Source: CAD feature listing. Evaluate the final solid. Frame: model axes, mm. A direction names the side the tool comes from. Coordinates: 2 decimals unless noted, no trailing zeros. Order: outer loops, then holes, each group sorted by start corner. A loop starts at its lowest first (then second) coordinate and runs counter-clockwise, first axis right, second up.
```python
from build123d import *

# Parameters (mm, degrees)
SKETCH1_W                                      = 25.4
SKETCH1_H                                      = 29
BOSS_EXTRUDE1_DEPTH                            = 8
SKETCH2_W                                      = 275
SKETCH2_H                                      = 29
BOSS_EXTRUDE2_DEPTH                            = 7
CBORE_FOR_8_SOCKET_HEAD_CAP_SCREW1_D           = 4.4958
CBORE_FOR_8_SOCKET_HEAD_CAP_SCREW1_DEPTH       = 18.649325414
CBORE_FOR_8_SOCKET_HEAD_CAP_SCREW1_CBORE_D     = 7.9375
CBORE_FOR_8_SOCKET_HEAD_CAP_SCREW1_CBORE_DEPTH = 4.1656
CBORE_FOR_8_SOCKET_HEAD_CAP_SCREW1_TIP         = 1.350674586
SKETCH5_W                                      = 64.25
SKETCH5_H                                      = 10.5
SKETCH5_W_2                                    = 109.45
SKETCH5_W_3                                    = 11.4
SKETCH5_W_4                                    = 6.7
CUT_EXTRUDE1_DEPTH                             = 10
FILLET1_R                                      = 3.9
FILLET2_R                                      = 3.5


with BuildPart() as part:
    # Sketch1 → Boss-Extrude1 (new body)
    with BuildSketch(Plane.XY):
        Rectangle(SKETCH1_W, SKETCH1_H)
    extrude(amount=BOSS_EXTRUDE1_DEPTH)

    # Sketch2 → Boss-Extrude2 (add)
    with BuildSketch(Plane.XY.offset(8)):
        with Locations((124.8, 0)):
            Rectangle(SKETCH2_W, SKETCH2_H)
    extrude(amount=BOSS_EXTRUDE2_DEPTH)

    # CBORE for #8 Socket Head Cap Screw1
    with Locations(Plane(origin=(-7.5, 7.5, 15), x_dir=(1, 0, 0), z_dir=(0, 0, 1))):
        with Locations((0, 0), (15, 0), (15, -15), (0, -15), (35.7, 0), (35.7, -15), (113.95, 0), (113.95, -15), (237.4, 0), (237.4, -15), (262.8, 0), (262.8, -15)):
            CounterBoreHole(CBORE_FOR_8_SOCKET_HEAD_CAP_SCREW1_D / 2, CBORE_FOR_8_SOCKET_HEAD_CAP_SCREW1_CBORE_D / 2, CBORE_FOR_8_SOCKET_HEAD_CAP_SCREW1_CBORE_DEPTH, depth=CBORE_FOR_8_SOCKET_HEAD_CAP_SCREW1_DEPTH)
            with Locations((0, 0, -(CBORE_FOR_8_SOCKET_HEAD_CAP_SCREW1_DEPTH + CBORE_FOR_8_SOCKET_HEAD_CAP_SCREW1_TIP / 2))):  # 118° drill point
                Cone(0, CBORE_FOR_8_SOCKET_HEAD_CAP_SCREW1_D / 2, CBORE_FOR_8_SOCKET_HEAD_CAP_SCREW1_TIP, mode=Mode.SUBTRACT)

    # Sketch5 → Cut-Extrude1 (cut)
    with BuildSketch(Plane.XY.offset(15)):
        with Locations((67.325, 9.25)):
            Rectangle(SKETCH5_W, SKETCH5_H)
        with Locations((168.175, 9.25)):
            Rectangle(SKETCH5_W_2, SKETCH5_H)
        with Locations((242.6, 9.25)):
            Rectangle(SKETCH5_W_3, SKETCH5_H)
        with Locations((17.85, 9.25)):
            Rectangle(SKETCH5_W_4, SKETCH5_H)
    cut_extrude1 = extrude(amount=-CUT_EXTRUDE1_DEPTH, mode=Mode.SUBTRACT)

    # Mirror1: Cut-Extrude1 across plane
    add(cut_extrude1.mirror(Plane.ZX), mode=Mode.SUBTRACT)

    # Fillet1
    # the kernel refuses this fillet: 3.9 mm, written as the material it takes off along each edge
    with BuildSketch(Plane(origin=(222.9, 4, 15), x_dir=(0, -1, 0), z_dir=(-1, 0, 0)), Plane(origin=(222.9, -4, 8), x_dir=(0, 1, 0), z_dir=(-1, 0, 0))) as fillet1_piece_1:
        with BuildLine():
            CenterArc((FILLET1_R, -FILLET1_R), FILLET1_R, 90, 90)
            Line((0, -FILLET1_R), (0, 0))
            Line((0, 0), (FILLET1_R, 0))
        make_face()
    extrude(amount=109.45, mode=Mode.SUBTRACT)
    with BuildSketch(Plane(origin=(248.3, 4, 15), x_dir=(0, -1, 0), z_dir=(-1, 0, 0)), Plane(origin=(248.3, -4, 8), x_dir=(0, 1, 0), z_dir=(-1, 0, 0))) as fillet1_piece_2:
        with BuildLine():
            CenterArc((FILLET1_R, -FILLET1_R), FILLET1_R, 90, 90)
            Line((0, -FILLET1_R), (0, 0))
            Line((0, 0), (FILLET1_R, 0))
        make_face()
    extrude(amount=11.4, mode=Mode.SUBTRACT)
    with BuildSketch(Plane(origin=(248.3, 4, 8), x_dir=(0, -1, 0), z_dir=(-1, 0, 0)), Plane(origin=(248.3, -4, 15), x_dir=(0, 1, 0), z_dir=(-1, 0, 0))) as fillet1_piece_3:
        with BuildLine():
            CenterArc((FILLET1_R, FILLET1_R), FILLET1_R, 180, 90)
            Line((0, FILLET1_R), (0, 0))
            Line((0, 0), (FILLET1_R, 0))
        make_face()
    extrude(amount=11.4, mode=Mode.SUBTRACT)
    with BuildSketch(Plane(origin=(222.9, -4, 15), x_dir=(0, 1, 0), z_dir=(-1, 0, 0)), Plane(origin=(222.9, 4, 8), x_dir=(0, -1, 0), z_dir=(-1, 0, 0))) as fillet1_piece_4:
        with BuildLine():
            CenterArc((FILLET1_R, FILLET1_R), FILLET1_R, 180, 90)
            Line((0, FILLET1_R), (0, 0))
            Line((0, 0), (FILLET1_R, 0))
        make_face()
    extrude(amount=109.45, mode=Mode.SUBTRACT)
    with BuildSketch(Plane(origin=(99.45, 4, 8), x_dir=(0, -1, 0), z_dir=(-1, 0, 0)), Plane(origin=(99.45, -4, 15), x_dir=(0, 1, 0), z_dir=(-1, 0, 0))) as fillet1_piece_5:
        with BuildLine():
            CenterArc((FILLET1_R, FILLET1_R), FILLET1_R, 180, 90)
            Line((0, FILLET1_R), (0, 0))
            Line((0, 0), (FILLET1_R, 0))
        make_face()
    extrude(amount=64.25, mode=Mode.SUBTRACT)
    with BuildSketch(Plane(origin=(99.45, 4, 15), x_dir=(0, -1, 0), z_dir=(-1, 0, 0)), Plane(origin=(99.45, -4, 8), x_dir=(0, 1, 0), z_dir=(-1, 0, 0))) as fillet1_piece_6:
        with BuildLine():
            CenterArc((FILLET1_R, -FILLET1_R), FILLET1_R, 90, 90)
            Line((0, -FILLET1_R), (0, 0))
            Line((0, 0), (FILLET1_R, 0))
        make_face()
    extrude(amount=64.25, mode=Mode.SUBTRACT)
    with BuildSketch(Plane(origin=(21.2, -4, 8), x_dir=(0, 1, 0), z_dir=(-1, 0, 0)), Plane(origin=(21.2, 4, 15), x_dir=(0, -1, 0), z_dir=(-1, 0, 0))) as fillet1_piece_7:
        with BuildLine():
            CenterArc((FILLET1_R, -FILLET1_R), FILLET1_R, 90, 90)
            Line((0, -FILLET1_R), (0, 0))
            Line((0, 0), (FILLET1_R, 0))
        make_face()
    extrude(amount=6.7, mode=Mode.SUBTRACT)
    with BuildSketch(Plane(origin=(21.2, -4, 15), x_dir=(0, 1, 0), z_dir=(-1, 0, 0)), Plane(origin=(21.2, 4, 8), x_dir=(0, -1, 0), z_dir=(-1, 0, 0))) as fillet1_piece_8:
        with BuildLine():
            CenterArc((FILLET1_R, FILLET1_R), FILLET1_R, 180, 90)
            Line((0, FILLET1_R), (0, 0))
            Line((0, 0), (FILLET1_R, 0))
        make_face()
    extrude(amount=6.7, mode=Mode.SUBTRACT)

    # Fillet2
    fillet2_edges = [part.edges().sort_by_distance(p)[0] for p in [
        (262.3, -14.5, 11.5),
        (14.5, 14.5, 11.5),
        (21.2, 14.5, 11.5),
        (262.3, 14.5, 11.5),
        (236.9, 14.5, 11.5),
        (248.3, 14.5, 11.5),
        (113.45, 14.5, 11.5),
        (222.9, 14.5, 11.5),
        (35.2, 14.5, 11.5),
        (99.45, 14.5, 11.5),
        (14.5, -14.5, 11.5),
        (21.2, -14.5, 11.5),
        (236.9, -14.5, 11.5),
        (248.3, -14.5, 11.5),
        (113.45, -14.5, 11.5),
        (222.9, -14.5, 11.5),
        (35.2, -14.5, 11.5),
        (99.45, -14.5, 11.5),
        (-12.7, -14.5, 7.5),
        (-12.7, 14.5, 7.5),
    ]]
    fillet(fillet2_edges, radius=FILLET2_R)


solid = part.part
```
1. Contact query for flat-ended pins moving along their axis: P1, Ø6.5, axis at x = 254.5, y = -7, coming from the +Z side; P2, Ø6, axis at x = 165.5, z = 12.5, coming from the +Y side; P3, Ø5, axis at x = -7.5, y = -7.5, coming from the +Z side; P4, Ø8, axis at x = 202, z = 7, coming from the -Y side. Output: stop coordinate, or through.
2. Section query D-D, the plane x = 152.5. Output: boundary loops of the cut face in (y, z).
3. Draft query along Y for faces 1 (the flat face through (28, 14.5, 11)), 2 (the cylindrical face through (251.335, -7.326, 12.946)), 3 (the flat face through (109, -1, 8)), 4 (the cylindrical face through (233.566, 5.98, 12.946)). Return one class per face: +Y half, -Y half, draft (parallel to the pull), parting line (faces both ways), or undercut.
4. Section query A-A, the plane x = 229.9. Output: boundary loops of the cut face in (y, z), plus the area to 3 significant figures.
5. Section query B-B, the plane z = 3.75. Output: boundary loops of the cut face in (x, y), plus the area to 3 significant figures.
6. Material intervals for line 1 along Y through (x, z) = (255.3, 14.1); line 2 along Y through (x, z) = (106.45, 9.95); line 3 along X through (y, z) = (3.5, 9.5), sorted ascending.
7. Access query for faces 5 (the cylindrical face through (28.49, 9.73, 9.4)), 6 (the cylindrical face through (31.866, -9.02, 12.946)). Directions: +Z, -Z, +X, -X, +Y, -Y. A direction counts if a zero-diameter tool reaches every point of the face in a straight line with its end or side. Return the directions, or none.
8. Section query C-C, the plane y = 7.5. Count the separate pieces of the cut face and the enclosed holes in it, plus the area to 3 significant figures.
Answer key:
1. P1: stops at z = 15
1. P2: stops at y = 3.98
1. P3: stops at z = 10.83
1. P4: stops at y = -3.89
2. outline: (-3.98, 11.5) arc R3.9 ccw to (-0.1, 8) - (0.1, 8) arc R3.9 ccw to (3.98, 11.5) arc R3.9 ccw to (0.1, 15) - (-0.1, 15) arc R3.9 ccw to start
3. face 1: +Y half
3. face 2: undercut
3. face 3: draft
3. face 4: undercut
4. outline: (-14.5, 8) - (-9.75, 8) - (-9.75, 10.83) - (-11.47, 10.83) - (-11.47, 15) - (-14.5, 15) - close; (-5.25, 8) - (5.25, 8) - (5.25, 10.83) - (3.53, 10.83) - (3.53, 15) - (-3.53, 15) - (-3.53, 10.83) - (-5.25, 10.83) - close; (9.75, 8) - (14.5, 8) - (14.5, 15) - (11.47, 15) - (11.47, 10.83) - (9.75, 10.83) - close
4. area: 111 mm2
5. outline: (-12.7, -11) arc R3.5 ccw to (-9.2, -14.5) - (11, -14.5) arc R3.5 ccw to (12.7, -14.06) - (12.7, 14.06) arc R3.5 ccw to (11, 14.5) - (-9.2, 14.5) arc R3.5 ccw to (-12.7, 11) - close; hole circle Ø4.5 at (-7.5, -7.5); hole circle Ø4.5 at (-7.5, 7.5); hole circle Ø4.5 at (7.5, -7.5); hole circle Ø4.5 at (7.5, 7.5)
5. area: 667 mm2
6. line 1: y = -14.5 to -11.47, -3.53 to 3.53, 11.47 to 14.5
6. line 2: y = -14.5 to -9.75, -5.25 to 5.25, 9.75 to 14.5
6. line 3: x = -12.7 to 14.5, 21.2 to 35.2, 99.45 to 113.45, 222.9 to 236.9, 248.3 to 262.3
7. face 5: +Z, -Z
7. face 6: +Z
8. separate pieces: 11
8. enclosed holes: 0
8. area: 439 mm2
